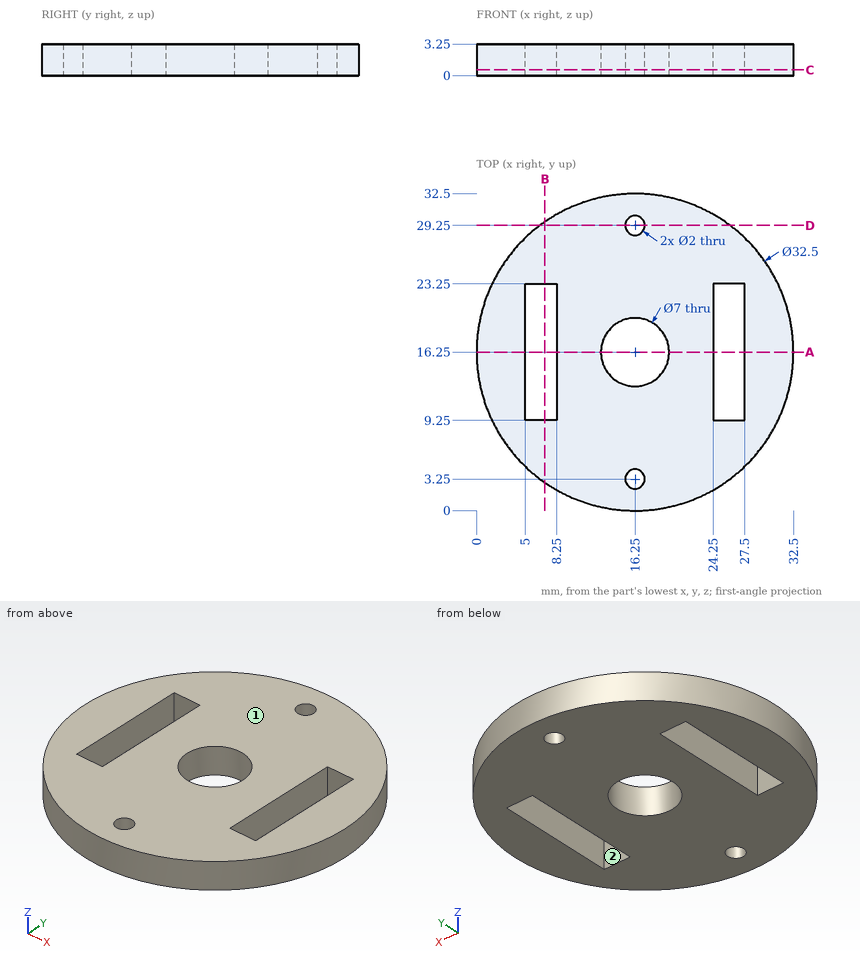
Can you work these out from the drawing? Everything is in mm from the part's minimum corner. A direction names the side the tool comes from. Round coordinates to 2 decimals unless told otherwise and drop trailing zeros. Order: outer loops, then holes, each group sorted by start corner. A loop starts at its lowest first (then second) coordinate and runs counter-clockwise, first axis right, second up. Notation, with made-up numbers: (60, 63.25) - (103, 63.25) arc R22 cw to (103, 83.25) - close; hole circle Ø1 at (39, 74). An arc over 180 degrees is marked (long way). Answer in a Markdown table with one row per item.
(1) Suppose I cut it at D-D, the plane y = 29.25. Please give me the cut outline in (x, z), plus the area to 3 significant figures.
From the geometry:
| item | result |
|---|---|
| outline | (6.5, 0) - (15.25, 0) - (15.25, 3.25) - (6.5, 3.25) - close; (17.25, 0) - (26, 0) - (26, 3.25) - (17.25, 3.25) - close |
| area | 56.9 mm2 |
(2) For P1, Ø1.6, axis at x = 7.5, z = 1, coming from the -Y side; P2, Ø1, axis at x = 22.5, z = 1.5, coming from the +Y side; P3, Ø1, axis at y = 19, z = 1.5, coming from the -X side, each with a flat end and sliding along its axis, tell me the tip position at first contact or that it passes through.
From the geometry:
| item | result |
|---|---|
| P1 | stops at y = 2.08 |
| P2 | stops at y = 31.45 |
| P3 | stops at x = 0.16 |
(3) Suppose I cut it at C-C, the plane z = 0.6. Please give me the cut outline in (x, y).
From the geometry:
| item | result |
|---|---|
| outline | circle Ø32.5 at (16.25, 16.25); hole (5, 9.25) - (8.25, 9.25) - (8.25, 23.25) - (5, 23.25) - close; hole circle Ø7 at (16.25, 16.25); hole circle Ø2 at (16.25, 3.25); hole circle Ø2 at (16.25, 29.25); hole (24.25, 9.25) - (27.5, 9.25) - (27.5, 23.25) - (24.25, 23.25) - close |
(4) Suppose I cut it at A-A, the plane y = 16.25. Please give me the cut outline in (x, z).
From the geometry:
| item | result |
|---|---|
| outline | (0, 0) - (5, 0) - (5, 3.25) - (0, 3.25) - close; (8.25, 0) - (12.75, 0) - (12.75, 3.25) - (8.25, 3.25) - close; (19.75, 0) - (24.25, 0) - (24.25, 3.25) - (19.75, 3.25) - close; (27.5, 0) - (32.5, 0) - (32.5, 3.25) - (27.5, 3.25) - close |
(5) Please list where these lines run through material, in increasing order: L1, parallel to Y at x = 16.25, z = 1.35; L2, parallel to X at y = 17.5, z = 2.5; L3, parallel to X at y = 20, z = 3. Write a range as from..to.
From the geometry:
| item | result |
|---|---|
| L1 | y = 0..2.25, 4.25..12.75, 19.75..28.25, 30.25..32.5 |
| L2 | x = 0.05..5, 8.25..12.98, 19.52..24.25, 27.5..32.45 |
| L3 | x = 0.44..5, 8.25..24.25, 27.5..32.06 |
(6) Suppose I cut it at B-B, the plane x = 7. Please give me the cut outline in (y, z), plus the area to 3 significant figures.
From the geometry:
| item | result |
|---|---|
| outline | (2.89, 0) - (9.25, 0) - (9.25, 3.25) - (2.89, 3.25) - close; (23.25, 0) - (29.61, 0) - (29.61, 3.25) - (23.25, 3.25) - close |
| area | 41.3 mm2 |
(7) Which directions (+Z, -Z, +X, -X, +Y, -Y) give clear straight access to the entire face, cutting with the end or side of a thin tool? Please do the marked faces 1 and 2.
From the geometry:
| item | result |
|---|---|
| face 1 | +Z, +X, -X, +Y, -Y |
| face 2 | +Z, -Z |
